```python
from build123d import *

# Parameters (mm, degrees)
SKETCH_W        = 18.3
SKETCH_H        = 12
SKETCH_R        = 1.5
SKETCH_R_2      = 1.6
PAD_DEPTH       = 5
SKETCH001_W     = 14
SKETCH001_H     = 12
SKETCH001_R     = 2.5
SKETCH001_R_2   = 1
POCKET_DEPTH    = 3.001
SKETCH002_R     = 3
POCKET001_DEPTH = 1
FILLET_R        = 3


with BuildPart() as part:
    # Sketch → Pad (new body)
    with BuildSketch(Plane.XY):
        with Locations((9.15, 6)):
            Rectangle(SKETCH_W, SKETCH_H)
        with Locations((9, 6)):
            Circle(SKETCH_R, mode=Mode.SUBTRACT)
        with Locations((2.5, 8)):
            Circle(SKETCH_R_2, mode=Mode.SUBTRACT)
    extrude(amount=PAD_DEPTH)

    # Sketch001 (on DatumPlane) → Pocket (cut, through all)
    with BuildSketch(Plane.XY.offset(2)):
        with Locations((12, 6)):
            Rectangle(SKETCH001_W, SKETCH001_H)
        with Locations((9, 6)):
            Circle(SKETCH001_R, mode=Mode.SUBTRACT)
        with Locations((14, 9.1)):
            Circle(SKETCH001_R_2, mode=Mode.SUBTRACT)
        with Locations((14, 2.9)):
            Circle(SKETCH001_R_2, mode=Mode.SUBTRACT)
    extrude(amount=POCKET_DEPTH, mode=Mode.SUBTRACT)

    # Sketch002 → Pocket001 (cut)
    with BuildSketch(Plane.XY):
        with Locations((2.5, 8)):
            Circle(SKETCH002_R)
        with Locations((9, 6)):
            Circle(SKETCH002_R)
    extrude(amount=POCKET001_DEPTH, mode=Mode.SUBTRACT)

    # Fillet
    fillet_edges = [part.edges().sort_by_distance(p)[0] for p in [
        (18.3, 0, 1),
    ]]
    fillet(fillet_edges, radius=FILLET_R)


with BuildPart() as part_1:
    # Body placement: moved
    add(part.part.moved(Location((-12, 0, 6.3))))


solid = part_1.part
```
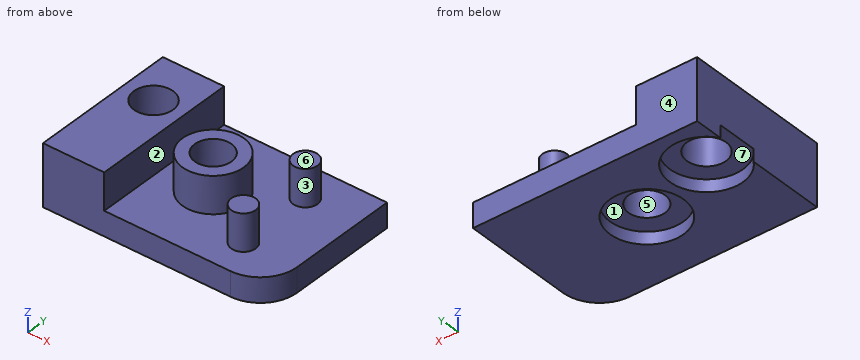
Input: part model. Units: mm. Frame: model coordinates. Face numbers are marked on the shaded views. A direction names the side the tool comes from. Coordinates: 2 decimals unless noted, no trailing zeros. Order: outer loops, then holes, each group sorted by start corner. A loop starts at its lowest first (then second) coordinate and runs counter-clockwise, first axis right, second up. Notation, with made-up numbers: (74.25, -15.75) - (106.25, -15.75) arc R12 cw to (106.25, -6.75) - close; hole circle Ø1 at (17.5, -36). An arc over 180 degrees is marked (long way). Return JSON: item names as keys, results as strings.
Q1. Access query for the marked faces 1, 2 and 3. Directions: +Z, -Z, +X, -X, +Y, -Y. A direction counts if a zero-diameter tool reaches every point of the face in a straight line with its end or side. Return the directions, or none.
The answers:
{"face 1": "-Z", "face 2": "+Z, +Y, -Y", "face 3": "+Z"}
Q2. First-contact query: pin 1 (1.5 mm diameter, centred on y = 8, z = 10.5, fed in from +X); pin 2 (1.8 mm diameter, centred on x = -2.5, y = 5.5, fed in from -Z); pin 3 (1 mm diameter, centred on x = 3, z = 9, fed in from -Y). Flat tips, straight axial feed; report the tip coordinate or a pass-through.
The answers:
{"pin 1": "stops at x = 2.94", "pin 2": "stops at z = 7.3", "pin 3": "stops at y = 2.03"}
Q3. Cut plane D-D (x = 2). Return loops of the section in (y, z).
The answers:
{"outline": "(0, 6.3) - (12, 6.3) - (12, 8.3) - (10.1, 8.3) - (10.1, 11.3) - (8.1, 11.3) - (8.1, 8.3) - (3.9, 8.3) - (3.9, 11.3) - (1.9, 11.3) - (1.9, 8.3) - (0, 8.3) - close"}
Q4. Cut plane C-C (y = 7.25). Return loops of the section in (x, z), then the cut area to 3 significant figures.
The answers:
{"outline": "(-12, 7.3) - (-10.91, 7.3) - (-10.91, 11.3) - (-12, 11.3) - close; (-8.09, 7.3) - (-6.6, 7.3) - (-6.6, 6.3) - (-5.73, 6.3) - (-5.73, 7.3) - (-3.83, 7.3) - (-3.83, 11.3) - (-5.17, 11.3) - (-5.17, 8.3) - (-7, 8.3) - (-7, 11.3) - (-8.09, 11.3) - close; (-2.17, 7.3) - (-0.27, 7.3) - (-0.27, 6.3) - (6.3, 6.3) - (6.3, 8.3) - (-0.83, 8.3) - (-0.83, 11.3) - (-2.17, 11.3) - close", "area": "35.8 mm2"}
Q5. Ray query, probe 1 along X at (y, z) = (8, 10.35); probe 2 along Y at (x, z) = (-9.5, 6.7); probe 3 along X at (y, z) = (6, 9.65). Return the intervals inside material, ascending.
The answers:
{"probe 1": "x = -12 to -11.1, -7.9 to -7, -4.5 to -1.5", "probe 2": "y = 0 to 5, 11 to 12", "probe 3": "x = -12 to -7, -5.5 to -4.5, -1.5 to -0.5"}
Q6. Cut plane B-B (x = -3). Return loops of the section in (y, z), then the cut area to 3 significant figures.
The answers:
{"outline": "(0, 6.3) - (3, 6.3) - (3, 7.3) - (4.5, 7.3) - (4.5, 11.3) - (3.5, 11.3) - (3.5, 8.3) - (0, 8.3) - close; (7.5, 7.3) - (9, 7.3) - (9, 6.3) - (12, 6.3) - (12, 8.3) - (8.5, 8.3) - (8.5, 11.3) - (7.5, 11.3) - close", "area": "21.0 mm2"}
Q7. Cut plane A-A (z = 8.8). Return loops of the section in (x, y).
The answers:
{"outline": "(-12, 0) - (-7, 0) - (-7, 12) - (-12, 12) - close; circle Ø5 at (-3, 6); circle Ø2 at (2, 2.9); circle Ø2 at (2, 9.1); hole circle Ø3.2 at (-9.5, 8); hole circle Ø3 at (-3, 6)"}
Q8. Draft query along Y for the marked faces 4, 5, 6 and 7. Return one class per face: +Y half, -Y half, draft (parallel to the pull), parting line (faces both ways), or undercut.
The answers:
{"face 4": "+Y half", "face 5": "undercut", "face 6": "draft", "face 7": "undercut"}
